from build123d import *

# Parameters (mm, degrees)
EXTRUDE_1_DEPTH   = 4
EXTRUDE_1_2_DEPTH = 4
EXTRUDE_1_3_DEPTH = 4
SKETCH_2_W        = 7
SKETCH_2_H        = 5
EXTRUDE_2_DEPTH   = 0.6
SKETCH_3_W        = 6
SKETCH_3_H        = 1.2
EXTRUDE_3_DEPTH   = 0.6
SKETCH_4_W        = 1
SKETCH_4_H        = 13
EXTRUDE_4_DEPTH   = 0.6
FILLET_1_R        = 0.5
SKETCH_5_W        = 1
SKETCH_5_H        = 0.6
EXTRUDE_5_DEPTH   = 1.2
FILLET_2_R        = 0.3
SKETCH_7_W        = 1
SKETCH_7_H        = 0.6
EXTRUDE_6_DEPTH   = 4


with BuildPart() as part:
    # Sketch 1 → Extrude 1 (new body)
    with BuildSketch(Plane(origin=(0, 0, 0), x_dir=(1, 0, 0), z_dir=(0, 1, 0))):
        with BuildLine():
            Line((-2.2, 1.7), (2.2, 1.7))
            ThreePointArc((2.2, 1.7), (2.694974747, 1.494974747), (2.9, 1))
            Line((2.9, 1), (2.9, -1))
            ThreePointArc((2.9, -1), (2.694974747, -1.494974747), (2.2, -1.7))
            Line((2.2, -1.7), (-2.2, -1.7))
            ThreePointArc((-2.2, -1.7), (-2.694974747, -1.494974747), (-2.9, -1))
            Line((-2.9, -1), (-2.9, 1))
            ThreePointArc((-2.9, 1), (-2.694974747, 1.494974747), (-2.2, 1.7))
        make_face()
    extrude(amount=EXTRUDE_1_DEPTH)



with BuildPart() as body_2:
    # Sketch 1 → Extrude 1 2 (new body)
    with BuildSketch(Plane(origin=(0, 0, 0), x_dir=(1, 0, 0), z_dir=(0, 1, 0))):
        with BuildLine():
            Line((-2.2, 7.528722779), (2.2, 7.528722779))
            ThreePointArc((2.2, 7.528722779), (2.694974747, 7.323697526), (2.9, 6.828722779))
            Line((2.9, 6.828722779), (2.9, 4.828722779))
            ThreePointArc((2.9, 4.828722779), (2.694974747, 4.333748032), (2.2, 4.128722779))
            Line((2.2, 4.128722779), (-2.2, 4.128722779))
            ThreePointArc((-2.2, 4.128722779), (-2.694974747, 4.333748032), (-2.9, 4.828722779))
            Line((-2.9, 4.828722779), (-2.9, 6.828722779))
            ThreePointArc((-2.9, 6.828722779), (-2.694974747, 7.323697526), (-2.2, 7.528722779))
        make_face()
    extrude(amount=EXTRUDE_1_2_DEPTH)


with BuildPart() as body_3:
    # Sketch 1 → Extrude 1 3 (new body)
    with BuildSketch(Plane(origin=(0, 0, 0), x_dir=(1, 0, 0), z_dir=(0, 1, 0))):
        with BuildLine():
            Line((-2.2, 13.349128593), (2.2, 13.349128593))
            ThreePointArc((2.2, 13.349128593), (2.694974747, 13.144103339), (2.9, 12.649128593))
            Line((2.9, 12.649128593), (2.9, 10.649128593))
            ThreePointArc((2.9, 10.649128593), (2.694974747, 10.154153846), (2.2, 9.949128593))
            Line((2.2, 9.949128593), (-2.2, 9.949128593))
            ThreePointArc((-2.2, 9.949128593), (-2.694974747, 10.154153846), (-2.9, 10.649128593))
            Line((-2.9, 10.649128593), (-2.9, 12.649128593))
            ThreePointArc((-2.9, 12.649128593), (-2.694974747, 13.144103339), (-2.2, 13.349128593))
        make_face()
    extrude(amount=EXTRUDE_1_3_DEPTH)


with BuildPart() as part_1:
    add(part.part)

    add(body_2.part)  # Extrude 2 merges body 2

    add(body_3.part)  # Extrude 2 merges body 3
    # Sketch 2 → Extrude 2 (add)
    with BuildSketch(Plane(origin=(0, 4, 0), x_dir=(1, 0, 0), z_dir=(0, 1, 0))):
        with Locations((0.036699987, 11.763062551)):
            Rectangle(SKETCH_2_W, SKETCH_2_H)
        with Locations((0.036699987, 5.863062551)):
            Rectangle(SKETCH_2_W, SKETCH_2_H)
        with Locations((0.036699987, -0.036937449)):
            Rectangle(SKETCH_2_W, SKETCH_2_H)
    extrude(amount=-EXTRUDE_2_DEPTH)

    # Sketch 3 → Extrude 3 (add)
    with BuildSketch(Plane(origin=(0, 4, 0), x_dir=(1, 0, 0), z_dir=(0, 1, 0))):
        with Locations((6.536699987, 11.763062551)):
            Rectangle(SKETCH_3_W, SKETCH_3_H)
        with Locations((6.536699987, 5.863062551)):
            Rectangle(SKETCH_3_W, SKETCH_3_H)
        with Locations((6.536699987, -0.036937449)):
            Rectangle(SKETCH_3_W, SKETCH_3_H)
    extrude(amount=-EXTRUDE_3_DEPTH)

    # Sketch 4 → Extrude 4 (add)
    with BuildSketch(Plane.XZ.offset(-3.4)):
        with Locations((9.036699987, -5.863062551)):
            Rectangle(SKETCH_4_W, SKETCH_4_H)
    extrude(amount=-EXTRUDE_4_DEPTH)

    # Fillet 1
    fillet_1_edges = [part_1.edges().sort_by_distance(p)[0] for p in [
        (3.536699987, 3.7, -11.163062551),
        (3.536699987, 3.7, -12.363062551),
        (3.536699987, 3.7, 0.636937449),
        (3.536699987, 3.7, -0.563062551),
        (3.536699987, 3.7, -5.263062551),
        (3.536699987, 3.7, -6.463062551),
    ]]
    fillet(fillet_1_edges, radius=FILLET_1_R)

    # Sketch 5 → Extrude 5 (add)
    with BuildSketch(Plane(origin=(0, 0, -12.363062551), x_dir=(-1, 0, 0), z_dir=(0, 0, -1))):
        with Locations((-9.036699987, 3.7)):
            Rectangle(SKETCH_5_W, SKETCH_5_H)
    extrude(amount=EXTRUDE_5_DEPTH)

    # Fillet 2
    fillet_2_edges = [part_1.edges().sort_by_distance(p)[0] for p in [
        (-2.9, 0, 0),
        (-2.694974747, 0, -1.494974747),
        (-2.694974747, 0, -13.144103339),
        (-2.9, 0, -11.649128593),
        (-2.694974747, 0, -10.154153846),
        (0, 0, -9.949128593),
        (2.694974747, 0, -10.154153846),
        (2.9, 0, -11.649128593),
        (2.694974747, 0, -13.144103339),
        (0, 0, -13.349128593),
        (0, 0, -1.7),
        (2.694974747, 0, -1.494974747),
        (2.9, 0, 0),
        (2.694974747, 0, 1.494974747),
        (-2.694974747, 0, -7.323697526),
        (-2.9, 0, -5.828722779),
        (-2.694974747, 0, -4.333748032),
        (0, 0, -4.128722779),
        (2.694974747, 0, -4.333748032),
        (2.9, 0, -5.828722779),
        (2.694974747, 0, -7.323697526),
        (0, 0, 1.7),
        (0, 0, -7.528722779),
        (-2.694974747, 0, 1.494974747),
    ]]
    fillet(fillet_2_edges, radius=FILLET_2_R)

    # Sketch 7 → Extrude 6 (add)
    with BuildSketch(Plane.XY.offset(0.636937449)):
        with Locations((9.036699987, 3.7)):
            Rectangle(SKETCH_7_W, SKETCH_7_H)
    extrude(amount=EXTRUDE_6_DEPTH)


solid = part_1.part
Design review of the part built by this model. Coordinates are the model's own, in mm. A direction names the side the tool comes from. Round coordinates to 2 decimals unless told otherwise and drop trailing zeros. Loops run counter-clockwise (first coordinate to the right, second up) from the corner with the lowest first, then second, coordinate; pieces in that order, holes last. Notation, with made-up numbers: (62, -15.5) -> (114, -15.5) arc R34 cw to (114, 23.5) -> close; hole circle Ø7 at (41, -26.75). An arc over 180 degrees is marked (long way). Use one line per item in the form item = value. Start each with the question number.
Q1. We need section B-B on x = 3.25. Give the boundary of the cut face in (y, z).
Q2. For pin 1 Ø2 at (y, z) = (2.5, -11.5) entering from +X; pin 2 Ø1.6 at (x, y) = (-0.5, 1.5) entering from +Z; pin 3 Ø0.7 at (x, y) = (-1, 3.5) entering from +Z, all flat-tipped, find the tip position at first contact; note any pin that passes through.
Q3. Wall thickness on line 1 along Z through (x, y) = (1.5, 2.2); line 2 along Z through (x, y) = (7.5, 3.55); line 3 along Y through (x, z) = (-2, 2): over which ranges is each line inside the solid? List them lowest first. Write a range as [from, to].
Q4. Draft analysis for pull direction Z (two halves, no side actions). For faces 1 (the face through (0, 2, -13.349)), 2 (the face through (2.9, 2, -6)), 3 (the face through (0, 2, -1.7)), state which applies: +Z half, -Z half, draft (parallel to the pull), parting line (faces both ways), or undercut.
Q5. Machinability: for faces 4 (the face through (2.9, 2, -12)), 5 (the face through (0, 2, 1.7)), 6 (the face through (-2.9, 2, -12)), 7 (the face through (0, 2, -4.129)), which of the approach directions +Z, -Z, +X, -X, +Y, -Y give a long, thin tool a straight path to every point of the face, cutting with its end or side? Answer none if there is none.
Q6. We need section A-A on z = -3.75. Give the boundary of the cut face in (x, y), then the cut area to 3 significant figures.
Q7. We need section D-D on z = -12. Give the boundary of the cut face in (x, y), then the cut area to 3 significant figures.
Q8. We need section C-C on y = 1.15. Give the boundary of the cut face in (x, z), then the cut area to 3 significant figures.
Calculated:
q1.outline = (3.4, -14.26) -> (4, -14.26) -> (4, -9.26) -> (3.4, -9.26) -> close; (3.4, -8.36) -> (4, -8.36) -> (4, -3.36) -> (3.4, -3.36) -> close; (3.4, -2.46) -> (4, -2.46) -> (4, 2.54) -> (3.4, 2.54) -> close
q2.pin_1 = 9.54
q2.pin_2 = 1.7
q2.pin_3 = 2.54
q3.line_1 = [-13.35, -9.95], [-7.53, -4.13], [-1.7, 1.7]
q3.line_2 = [-12.36, -11.16], [-6.46, -5.26], [-0.56, 0.64]
q3.line_3 = [3.4, 4]
q4.face_1 = -Z half
q4.face_2 = draft
q4.face_3 = undercut
q5.face_4 = +Z, -Z, +X, -Y
q5.face_5 = +Z, +X, -X, -Y
q5.face_6 = +Z, -Z, -X, -Y
q5.face_7 = +X, -X, -Y
q6.outline = (-3.46, 3.4) -> (3.54, 3.4) -> (3.54, 4) -> (-3.46, 4) -> close; (8.54, 3.4) -> (9.54, 3.4) -> (9.54, 4) -> (8.54, 4) -> close
q6.area = 4.80 mm²
q7.outline = (-3.46, 3.4) -> (-2.9, 3.4) -> (-2.9, 0.3) arc R0.3 ccw to (-2.6, 0) -> (2.6, 0) arc R0.3 ccw to (2.9, 0.3) -> (2.9, 3.4) -> (9.54, 3.4) -> (9.54, 4) -> (-3.46, 4) -> close
q7.area = 27.5 mm²
q8.outline = (-2.9, -12.65) arc R0.7 ccw to (-2.2, -13.35) -> (2.2, -13.35) arc R0.7 ccw to (2.9, -12.65) -> (2.9, -10.65) arc R0.7 ccw to (2.2, -9.95) -> (-2.2, -9.95) arc R0.7 ccw to (-2.9, -10.65) -> close; (-2.9, -6.83) arc R0.7 ccw to (-2.2, -7.53) -> (2.2, -7.53) arc R0.7 ccw to (2.9, -6.83) -> (2.9, -4.83) arc R0.7 ccw to (2.2, -4.13) -> (-2.2, -4.13) arc R0.7 ccw to (-2.9, -4.83) -> close; (-2.9, -1) arc R0.7 ccw to (-2.2, -1.7) -> (2.2, -1.7) arc R0.7 ccw to (2.9, -1) -> (2.9, 1) arc R0.7 ccw to (2.2, 1.7) -> (-2.2, 1.7) arc R0.7 ccw to (-2.9, 1) -> close
q8.area = 57.9 mm²
